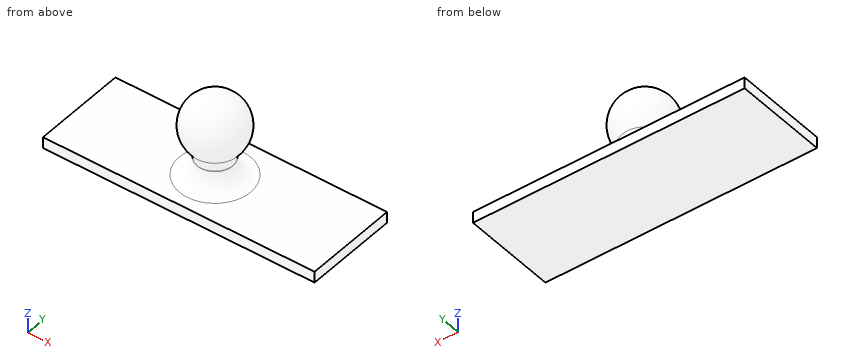
```python
from build123d import *

# Parameters (mm, degrees)
F0_W     = 77.47
F0_H     = 26.67
F1_DEPTH = 3.175
F2_R     = 5.08
F3_DEPTH = 14.525168
F6_R     = 5.08


with BuildPart() as f1:
    # F0 (on Top) → F1 (new body)
    with BuildSketch(Plane.XY):
        Rectangle(F0_W, F0_H)
    extrude(amount=F1_DEPTH)

    # F2 (on face) → F3 (join)
    with BuildSketch(Plane.XY.offset(3.175)):
        Circle(F2_R)
    extrude(amount=F3_DEPTH)

    # F4 (on Front) → F5 (revolve)
    with BuildSketch(Plane.XZ):
        with BuildLine():
            Line((0, 26.399668), (0, 9.000668))
            ThreePointArc((0, 9.000668), (8.6995, 17.700168), (0, 26.399668))
        make_face()
    revolve(axis=Axis((0, 0, 17.700168), (0, 0, -1)))

    # F6
    f6_edges = [f1.edges().sort_by_distance(p)[0] for p in [
        (-5.08, 0, 3.175),
        (-5.08, 0, 10.637951),
    ]]
    fillet(f6_edges, radius=F6_R)


solid = f1.part
```
Work out the finished part from the listing and answer in its coordinate system (mm). Give positions to 0.01 mm unless a question says otherwise; leave off trailing zeros. Loops run counter-clockwise (first coordinate to the right, second up) from the corner with the lowest first, then second, coordinate; pieces in that order, holes last. Notation, with made-up numbers: (-19.5, -38) -> (-6.5, -38) arc R26 cw to (-6.5, -18) -> close; hole circle Ø7 at (-14.75, 12). An arc over 180 degrees is marked (long way). Put each result on its own line as item: value. Start each with the question number.
Item 1: The part is cut by section A-A (x = 27). Give the vertices of the cut face in (y, z) (3 decimals).
Item 2: The part is cut by section C-C (z = 23.5). Give the vertices of the cut face in (x, y).
Item 3: The part is cut by section B-B (z = 6). Give the vertices of the cut face in (x, y).
Item 4: Each of these flat-tipped pins is pushed along its axis until it touches: P1, Ø1, axis at x = 12, y = -4.5, coming from the +Z side (3 decimals); P2, Ø1.5, axis at x = 0.5, z = 8, coming from the -Y side; P3, Ø6, axis at x = 18.5, y = 1.5, coming from the -Z side; P4, Ø1.5, axis at y = -4.5, z = 7.5, coming from the -X side. Where does it stop, or does it pass through?
Item 5: Find the intervals of material crossed by L1, parallel to Z at x = -19, y = -2.75 (3 decimals); L2, parallel to Z at x = 2, y = -5.25; L3, parallel to Y at x = -1.5, z = 15.5, in increasing order. Write a range as [from, to].
Answers below:
1. outline: (-13.335, 0) -> (13.335, 0) -> (13.335, 3.175) -> (-13.335, 3.175) -> close
2. outline: circle Ø12.97 at (0, 0)
3. outline: circle Ø11.22 at (0, 0)
4. P1: z = 3.175
4. P2: y = -5.17
4. P3: z = 0
4. P4: x = -3.53
5. L1: [0, 3.175]
5. L2: [0, 5.98], [10.67, 24.34]
5. L3: [-8.28, 8.28]
